from build123d import *

# Parameters (mm, degrees)
F0_W     = 1450
F0_H     = 125
F0_W_2   = 1400
F0_H_2   = 75
F1_DEPTH = 331
F2_W     = 1400
F2_H     = 281
F3_DEPTH = 377
F4_W     = 281
F4_H     = 75
F5_DEPTH = 1538


with BuildPart() as f1:
    # F0 (on Front) → F1 (new body)
    with BuildSketch(Plane.XZ):
        with Locations((-725, 62.5)):
            Rectangle(F0_W, F0_H)
        with Locations((-725, 62.5)):
            Rectangle(F0_W_2, F0_H_2, mode=Mode.SUBTRACT)
    extrude(amount=-F1_DEPTH)

    # F2 (on Top) → F3 (cut)
    with BuildSketch(Plane.XY):
        with Locations((-725, 165.5)):
            Rectangle(F2_W, F2_H)
    extrude(amount=F3_DEPTH, mode=Mode.SUBTRACT)

    # F4 (on Right) → F5 (cut)
    with BuildSketch(Plane.YZ):
        with Locations((165.5, 62.5)):
            Rectangle(F4_W, F4_H)
    extrude(amount=-F5_DEPTH, mode=Mode.SUBTRACT)


solid = f1.part
The model under review builds one solid part; all positions refer to its coordinate system, in mm. A direction names the side the tool comes from. Round coordinates to 2 decimals unless told otherwise and drop trailing zeros. Order: outer loops, then holes, each group sorted by start corner. A loop starts at its lowest first (then second) coordinate and runs counter-clockwise, first axis right, second up. Notation, with made-up numbers: (-7.75, 65) -> (4.25, 65) arc R15 ccw to (4.25, 69) -> close; hole circle Ø1 at (-12.75, -20.75). An arc over 180 degrees is marked (long way). Write item = value, one per line. Start each with the question number.
Item 1: For line 1 along Z through (x, y) = (-895, 14); line 2 along Y through (x, z) = (-1056, 108.5); line 3 along X through (y, z) = (64, 23.5), list the stretches that pass through material, from the lowest coordinate up.
Item 2: Consider section A-A on z = 43.5. Write out the cut boundary in (x, y).
Item 3: Consider section B-B on y = 200.5. Write out the cut boundary in (x, z), plus the area to 3 significant figures.
Item 4: Mouldability with a two-part tool opening along Y and no side actions: class faces 4 (the face through (-735, 331, 105)), 5 (the face through (-1450, 163, 103)), 6 (the face through (-25, 164, 112)) as released by +Y, released by -Y, zero draft, split by the parting line, or undercut.
Item 5: For faces 1 (the face through (-12, 164, 100)), 2 (the face through (-735, 25, 112)), 3 (the face through (-735, 318, 25)), list the 3-axis set-ups (+Z, -Z, +X, -X, +Y, -Y) from which the entire face can be reached by the end or side of a thin tool; tool diameter is ignored.
Conclusion:
q1.line_1 = 0 to 25, 100 to 125
q1.line_2 = 0 to 25, 306 to 331
q1.line_3 = -1450 to -1425, -25 to 0
q2.outline = (-1450, 0) -> (-1425, 0) -> (-1425, 25) -> (-1450, 25) -> close; (-1450, 306) -> (-1425, 306) -> (-1425, 331) -> (-1450, 331) -> close; (-25, 0) -> (0, 0) -> (0, 25) -> (-25, 25) -> close; (-25, 306) -> (0, 306) -> (0, 331) -> (-25, 331) -> close
q3.outline = (-1450, 0) -> (-1425, 0) -> (-1425, 25) -> (-1450, 25) -> close; (-1450, 100) -> (-1425, 100) -> (-1425, 125) -> (-1450, 125) -> close; (-25, 0) -> (0, 0) -> (0, 25) -> (-25, 25) -> close; (-25, 100) -> (0, 100) -> (0, 125) -> (-25, 125) -> close
q3.area = 2,500 mm2
q4.face_4 = released by +Y
q4.face_5 = zero draft
q4.face_6 = undercut
q5.face_1 = +X, -X
q5.face_2 = +Z, -Z
q5.face_3 = +Y, -Y
